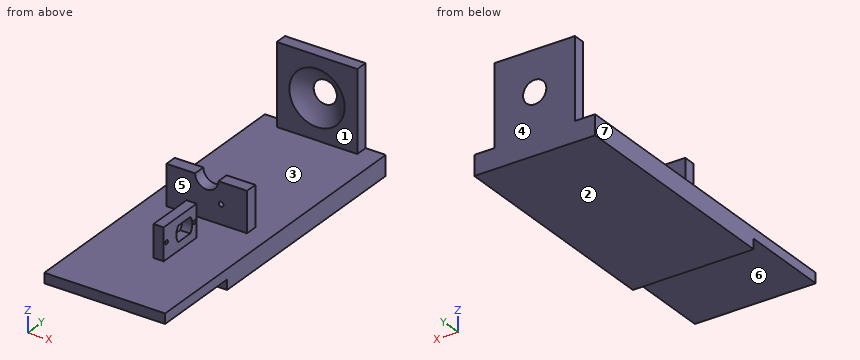
```python
from build123d import *

# Parameters (mm, degrees)
F1_DEPTH  = 38.1
F0_W      = 30.48
F0_H      = 20.32
F0_R      = 1.27
F2_DEPTH  = 6.35
F0_W_2    = 7.62
F0_H_2    = 25.4
F3_DEPTH  = 25.4
F0_H_3    = 50.8
F4_DEPTH  = 25.4
F7_R      = 7.3205
F8_DEPTH  = 109.221
F9_R      = 1.464692
F10_DEPTH = 25.4


with BuildPart() as f1:
    # F0 (on Right) → F1 (new body, symmetric)
    with BuildSketch(Plane.YZ):
        Polygon((-56.604175, 6.311384), (-101.6, 6.311384), (-101.6, 0), (-44.45, 0), (-44.45, -6.311384), (101.6, -6.311384), (101.6, 6.311384), (93.98, 6.311384), (0, 6.311384), (-7.62, 6.311384), (-26.124175, 6.311384), align=None)
    extrude(amount=F1_DEPTH, both=True)

    # F0 (on Right) → F2 (join)
    with BuildSketch(Plane.YZ):
        with Locations((-41.364175, 16.471384)):
            Rectangle(F0_W, F0_H)
        with Locations((-53.956132, 16.471384)):
            Circle(F0_R, mode=Mode.SUBTRACT)
        with BuildLine():
            ThreePointArc((-32.089956, 21.411047), (-30.188175, 16.471384), (-32.089956, 11.531721))
            Line((-32.089956, 11.531721), (-43.018393, 11.531721))
            ThreePointArc((-43.018393, 11.531721), (-44.920175, 16.471384), (-43.018393, 21.411047))
            Line((-43.018393, 21.411047), (-32.089956, 21.411047))
        make_face(mode=Mode.SUBTRACT)
        with Locations((-27.746813, 16.471384)):
            Circle(F0_R, mode=Mode.SUBTRACT)
    extrude(amount=F2_DEPTH)

    # F0 (on Right) → F3 (join, symmetric)
    with BuildSketch(Plane.YZ):
        with Locations((-3.81, 19.011384)):
            Rectangle(F0_W_2, F0_H_2)
    extrude(amount=F3_DEPTH, both=True)

    # F0 (on Right) → F4 (join, symmetric)
    with BuildSketch(Plane.YZ):
        with Locations((97.79, 31.711384)):
            Rectangle(F0_W_2, F0_H_3)
    extrude(amount=F4_DEPTH, both=True)

    # F5 (on Right) → F6 (revolve, cut)
    with BuildSketch(Plane.YZ):
        with BuildLine():
            Line((81.28, 10.121384), (81.28, 53.301384))
            ThreePointArc((81.28, 53.301384), (59.69, 31.711384), (81.28, 10.121384))
        make_face()
    revolve(axis=Axis((0, 81.28, 31.711384), (0, 0, -1)), mode=Mode.SUBTRACT)

    # F7 (on face) → F8 (cut, through all)
    with BuildSketch(Plane.XZ.offset(7.62)):
        with Locations((0, 31.711384)):
            Circle(F7_R)
    extrude(amount=-F8_DEPTH, mode=Mode.SUBTRACT)

    # F9 (on face) → F10 (cut)
    with BuildSketch(Plane.XZ.offset(7.62)):
        with Locations((9.084395, 18.466871)):
            Circle(F9_R)
    extrude(amount=-F10_DEPTH, mode=Mode.SUBTRACT)


solid = f1.part
```
Check sheet for the modelled part. Datum: model origin and axes. Units: mm. Face numbers are marked on the shaded views. A direction names the side the tool comes from. Round coordinates to 2 decimals unless told otherwise and drop trailing zeros. Write each loop counter-clockwise with the first axis right and the second up, starting at its lowest first coordinate (ties: lowest second). Pieces come first, ordered by that corner, then holes. Notation, with made-up numbers: (-16, 29.25) -> (21, 29.25) arc R16 cw to (21, 45.25) -> close; hole circle Ø7 at (-1, -33). An arc over 180 degrees is marked (long way). One line per question, with ' | ' between items. Start each with the question number.
1. Scan lines: line 1 along Y through (x, z) = (-1, 13); line 2 along Z through (x, y) = (-28, -33); line 3 along Y through (x, z) = (11, 30.5). Record each from-to range of solid material in increasing order. Write a range as from..to.
2. Sectioned sample at D-D, the plane x = 14.5. Record the cut outline in (y, z).
3. Sectioned sample at C-C, the plane y = -19. Record the cut outline in (x, z).
4. Depth check by flat-ended pin: pin 1 (1.5 mm diameter, centred on x = -27.5, y = 29, fed in from +Z); pin 2 (13 mm diameter, centred on x = 0, z = 31.71, fed in from +Y); pin 3 (1.5 mm diameter, centred on y = -8, z = 12.5, fed in from -X). Enter the tip coordinate at first touch or a pass-through.
5. Release check for a two-part mould opening along Y. For the marked faces 1, 2, 3 and 4 record: +Y half, -Y half, draft (parallel to the pull), parting line (faces both ways), or undercut.
6. Set-up check for the marked faces 5, 6 and 7: record each of +Z, -Z, +X, -X, +Y, -Y from which the full face is reachable in a straight line by a thin tool's end or side.
7. Sectioned sample at B-B, the plane x = 30.5. Record the cut outline in (y, z), then the cut area to 3 significant figures.
Taken from the geometry:
1) line 1: y = -7.62..0, 93.98..101.6 | line 2: z = -6.31..6.31 | line 3: y = -7.62..0, 99.82..101.6
2) outline: (-101.6, 0) -> (-44.45, 0) -> (-44.45, -6.31) -> (101.6, -6.31) -> (101.6, 57.11) -> (93.98, 57.11) -> (93.98, 41.44) arc R16 cw to (93.98, 21.99) -> (93.98, 6.31) -> (0, 6.31) -> (0, 31.71) -> (-7.62, 31.71) -> (-7.62, 6.31) -> (-101.6, 6.31) -> close
3) outline: (-38.1, -6.31) -> (38.1, -6.31) -> (38.1, 6.31) -> (-38.1, 6.31) -> close
4) pin 1: stops at z = 6.31 | pin 2: stops at y = -26.12 | pin 3: stops at x = -25.4
5) face 1: undercut | face 2: draft | face 3: undercut | face 4: +Y half
6) face 5: +Z, +X, -X | face 6: -Z, +X, -X, -Y | face 7: +Z, -Z, -X, +Y, -Y
7) outline: (-101.6, 0) -> (-44.45, 0) -> (-44.45, -6.31) -> (101.6, -6.31) -> (101.6, 6.31) -> (-101.6, 6.31) -> close | area: 2,200 mm^2
